from build123d import *

# Parameters (mm, degrees)
SKETCH_W   = 30
SKETCH_H   = 30
SKETCH_W_2 = 24
SKETCH_H_2 = 24
PAD_DEPTH  = 1000
FILLET_R   = 1


with BuildPart() as part:
    # Sketch → Pad (new body)
    with BuildSketch(Plane.XY):
        with Locations((15, 15)):
            Rectangle(SKETCH_W, SKETCH_H)
        with Locations((15, 15)):
            Rectangle(SKETCH_W_2, SKETCH_H_2, mode=Mode.SUBTRACT)
    extrude(amount=PAD_DEPTH)

    # Fillet
    fillet_edges = [part.edges().sort_by_distance(p)[0] for p in [
        (30, 0, 500),
        (0, 0, 500),
        (0, 30, 500),
        (30, 30, 500),
    ]]
    fillet(fillet_edges, radius=FILLET_R)


solid = part.part
Could you check a few things on this model? Use its own coordinates, in mm. A direction names the side the tool comes from. Coordinates: 2 decimals unless noted, no trailing zeros. Order: outer loops, then holes, each group sorted by start corner. A loop starts at its lowest first (then second) coordinate and runs counter-clockwise, first axis right, second up.
Q1. Thinking about a two-plate mould opening in Y: for faces 3 (the flat face through (15, 3, 493)), 4 (the flat face through (15, 30, 493)), 5 (the flat face through (0, 15, 493)), which applies, released by +Y, released by -Y, zero draft, split by the parting line, or undercut?
Q2. Suppose I cut it at A-A on x = 13.5. Please give me the cut outline in (y, z), and give its area (3 significant figures).
Q3. Suppose I cut it at C-C on z = 605. Please give me the cut outline in (x, y).
Q4. Please list where this line runs through material, in increasing order: L1, parallel to Y at x = 23.5, z = 676.5.
Q5. Which directions (+Z, -Z, +X, -X, +Y, -Y) give clear straight access to the entire face, cutting with the end or side of a thin tool? Please do faces 1 (the flat face through (30, 15, 493)), 2 (the flat face through (27, 15, 493)).
Answer:
1. face 3: undercut
1. face 4: released by +Y
1. face 5: zero draft
2. outline: (0, 0) - (3, 0) - (3, 1000) - (0, 1000) - close; (27, 0) - (30, 0) - (30, 1000) - (27, 1000) - close
2. area: 6,000 mm2
3. outline: (0, 1) arc R1 ccw to (1, 0) - (29, 0) arc R1 ccw to (30, 1) - (30, 29) arc R1 ccw to (29, 30) - (1, 30) arc R1 ccw to (0, 29) - close; hole (3, 3) - (27, 3) - (27, 27) - (3, 27) - close
4. L1: y = 0 to 3, 27 to 30
5. face 1: +Z, -Z, +X, +Y, -Y
5. face 2: +Z, -Z
